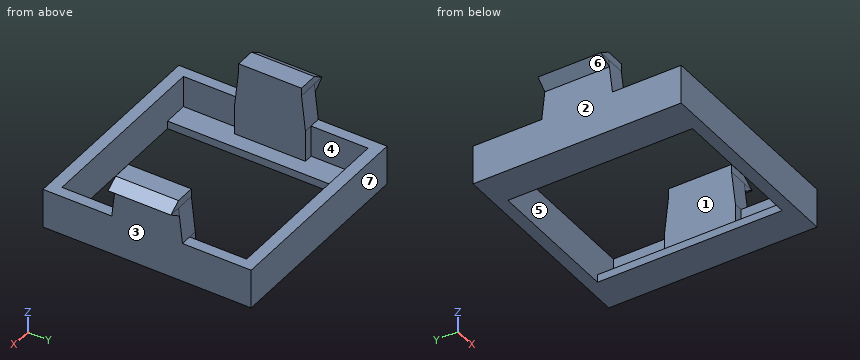
```python
from build123d import *

# Parameters (mm, degrees)
F0_W          = 26.5
F0_H          = 26.5
F0_W_2        = 23.7
F0_H_2        = 23.5
F1_DEPTH      = 5
F2_W          = 26.5
F2_H          = 26.5
F2_W_2        = 17.5
F2_H_2        = 23.5
F3_DEPTH      = 1
F5_DEPTH      = 2.5
F6_W          = 8
F6_H          = 1
F7_DEPTH      = 1.5
F9_DEPTH      = 25
F9_DEPTH_BACK = 25


with BuildPart() as f1:
    # F0 (on Top) → F1 (new body)
    with BuildSketch(Plane.XY):
        Rectangle(F0_W, F0_H)
        Rectangle(F0_W_2, F0_H_2, mode=Mode.SUBTRACT)
    extrude(amount=F1_DEPTH)

    # F2 (on Top) → F3 (join)
    with BuildSketch(Plane.XY):
        Rectangle(F2_W, F2_H)
        Rectangle(F2_W_2, F2_H_2, mode=Mode.SUBTRACT)
    extrude(amount=F3_DEPTH)

    # F4 (on face) → F5 (join)
    with BuildSketch(Plane(origin=(-13.25, 0, 0), x_dir=(0, -1, 0), z_dir=(-1, 0, 0))):
        Polygon((4.5, 5), (0, 5), (-4.5, 5), (-4.5, 0), (4.5, 0), align=None)
        Polygon((-4.5, 5), (0, 5), (0, 9.5), (-4, 9.5), align=None)
        Polygon((0, 9.5), (0, 5), (4.5, 5), (4, 9.5), align=None)
        Polygon((-4, 9.5), (0, 9.5), (4, 9.5), (4, 10.5), (-4, 10.5), align=None)
    extrude(amount=-F5_DEPTH)

    # F6 (on face) → F7 (join)
    with BuildSketch(Plane(origin=(-13.25, 0, 0), x_dir=(0, -1, 0), z_dir=(-1, 0, 0))):
        Polygon((-4, 9.5), (-4.110432, 8.506116), (4.110432, 8.506116), (4, 9.5), align=None)
        with Locations((0, 10)):
            Rectangle(F6_W, F6_H)
    extrude(amount=F7_DEPTH)

    # F8 (on Front) → F9 (cut, two sides)
    with BuildSketch(Plane.XZ) as f9_sk:
        Polygon((-14.75, 8.506116), (-13.25, 8.506116), (-14.75, 9.5), align=None)
        Polygon((-14.75, 10.5), (-14.75, 9.5), (-13.25, 10.5), align=None)
    extrude(amount=F9_DEPTH, mode=Mode.SUBTRACT)
    extrude(f9_sk.sketch, amount=-F9_DEPTH_BACK, mode=Mode.SUBTRACT)

    # F10: F1 across plane


with BuildPart() as f1_1:
    add(f1.part)
    add(f1.part.mirror(Plane.YZ))


solid = f1_1.part
```
Read the model definition and answer for the solid it produces. Units are mm, in the model's axes. Face numbers are marked on the shaded views. A direction names the side the tool comes from. Round coordinates to 2 decimals unless told otherwise and drop trailing zeros. Write each loop counter-clockwise with the first axis right and the second up, starting at its lowest first coordinate (ties: lowest second). Pieces come first, ordered by that corner, then holes. Notation, with made-up numbers: M 18,73 L 54,73 A33 ccw 54,102 Z; hole C 71.5,20 d7. An arc over 180 degrees is marked long. One line per item, written item: value.
Q1. Straight lines are drawn through the part: line 1 (Y direction, x = -11.75, z = 2.25); line 2 (X direction, y = -0.5, z = 3); line 3 (X direction, y = -5.5, z = 3.75). For each, find the intervals that lie inside material, in ascending order. Write a range as [from, to].
Data:
line 1: [-13.25, -11.75], [-4.5, 4.5], [11.75, 13.25]
line 2: [-13.25, -10.75], [10.75, 13.25]
line 3: [-13.25, -11.85], [11.85, 13.25]
Q2. For a pull along Y with two mould halves and no side action, classify the marked faces 4, 5, 6 and 7 as +Y half, -Y half, draft (parallel to the pull), parting line (faces both ways), or undercut.
Data:
face 4: undercut
face 5: undercut
face 6: draft
face 7: +Y half
Q3. Find section D-D on z = 3.25. Write down the section's boundary in (x, y), plus the area to 3 significant figures.
Data:
outline: M -13.25,-13.25 L 13.25,-13.25 L 13.25,13.25 L -13.25,13.25 Z; hole M -11.85,-11.75 L 11.85,-11.75 L 11.85,-4.5 L 10.75,-4.5 L 10.75,4.5 L 11.85,4.5 L 11.85,11.75 L -11.85,11.75 L -11.85,4.5 L -10.75,4.5 L -10.75,-4.5 L -11.85,-4.5 Z
area: 165 mm2
Q4. Find section C-C on z = 7.25. Write down the section's boundary in (x, y).
Data:
outline: M -13.25,-4.25 L -10.75,-4.25 L -10.75,4.25 L -13.25,4.25 Z; M 10.75,-4.25 L 13.25,-4.25 L 13.25,4.25 L 10.75,4.25 Z
Q5. Which of the six approach directions +Z, -Z, +X, -X, +Y, -Y give full straight-line access (tool end or side, diameter ignored) to the marked faces 1, 2 and 3?
Data:
face 1: +Z
face 2: -Z, -X, +Y, -Y
face 3: -Z, +X, +Y, -Y
Q6. Find section A-A on y = 3. Write down the section's boundary in (x, z), plus the area to 3 significant figures.
Data:
outline: M -14.75,9.5 L -13.25,8.51 L -13.25,0 L -8.75,0 L -8.75,1 L -10.75,1 L -10.75,10.5 L -13.25,10.5 Z; M 8.75,0 L 13.25,0 L 13.25,8.51 L 14.75,9.5 L 13.25,10.5 L 10.75,10.5 L 10.75,1 L 8.75,1 Z
area: 59.5 mm2
Q7. Flat-ended cylindrical pins translate along their axes: pin 1 Ø1.1 at (y, z) = (-1.5, 0.5) entering from -X; pin 2 Ø0.8 at (x, z) = (-13.5, 10) entering from -Y; pin 3 Ø0.5 at (x, z) = (-12, 10) entering from +Y. Find the tip coordinate at first contact, or state that the pin passes through.
Data:
pin 1: x = -13.25
pin 2: y = -4
pin 3: y = 4
Q8. Find section B-B on x = -4. Write down the section's boundary in (y, z).
Data:
outline: M -13.25,0 L -11.75,0 L -11.75,5 L -13.25,5 Z; M 11.75,0 L 13.25,0 L 13.25,5 L 11.75,5 Z
